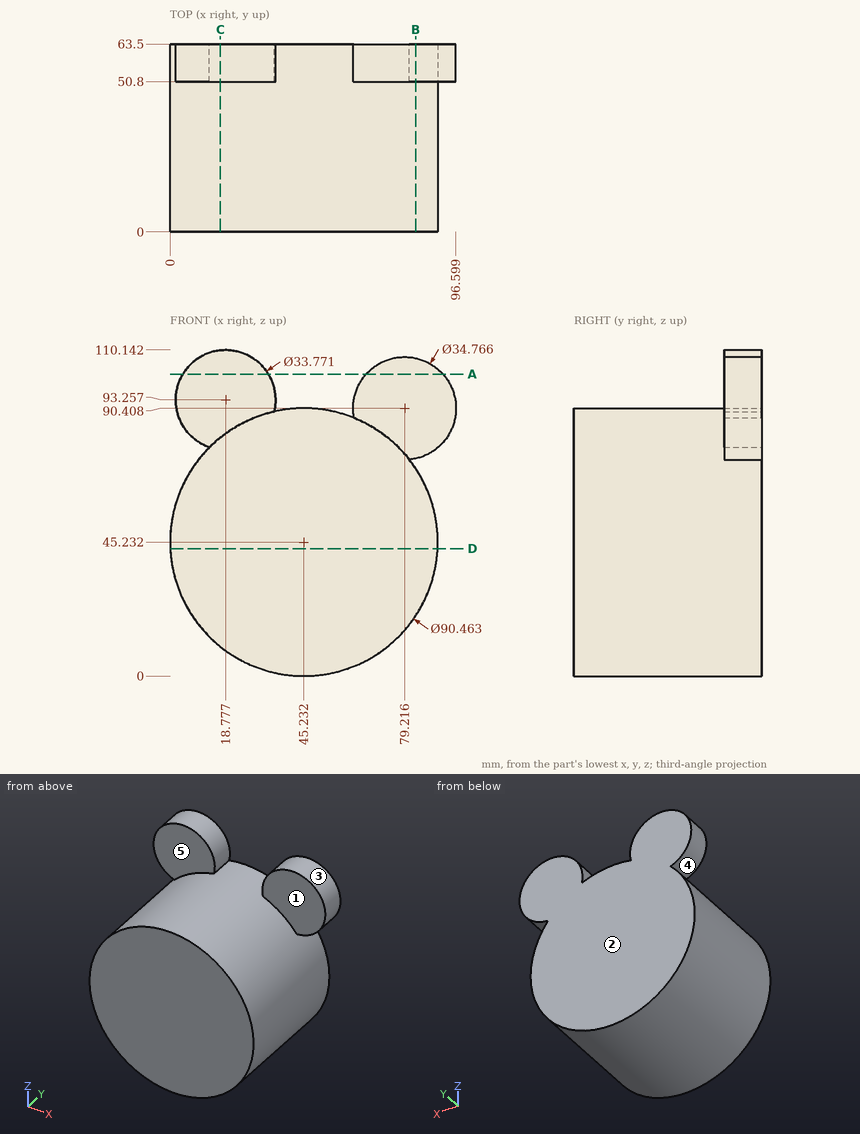
Geometry: see drawing. Coordinates: mm, zero at the bounding-box minimum. A direction names the side the tool comes from. Give positions to 0.01 mm unless a question says otherwise; leave off trailing zeros. Order: outer loops, then holes, each group sorted by start corner. A loop starts at its lowest first (then second) coordinate and runs counter-clockwise, first axis right, second up.
1. Pin query (flat end, axial travel): pin 1 Ø17.5 at (x, z) = (78, 93.5) entering from -Y; pin 2 Ø5 at (x, z) = (53.5, 80.5) entering from -Y; pin 3 Ø8 at (x, y) = (83, 12.5) entering from -Z; pin 4 Ø8 at (x, y) = (86.5, 47) entering from +Z. Return the tip coordinate at first contact, or that it passes through.
Computed:
pin 1: stops at y = 50.8
pin 2: stops at y = 0
pin 3: stops at z = 15.14
pin 4: stops at z = 106.71
2. Cut plane A-A (z = 102). Return loops of the section in (x, y).
Computed:
outline: (4.33, 50.8) - (33.22, 50.8) - (33.22, 63.5) - (4.33, 63.5) - close; (66.26, 50.8) - (92.17, 50.8) - (92.17, 63.5) - (66.26, 63.5) - close
3. Line query: probe 1 along Y at (x, z) = (83, 100); probe 2 along Z at (x, y) = (64.5, 34) (1 decimal); probe 3 along X at (y, z) = (47, 49.5). Output: solid intervals per line, ascending.
Computed:
probe 1: y = 50.8 to 63.5
probe 2: z = 4.3 to 86.2
probe 3: x = 0.2 to 90.26
4. Cut plane B-B (x = 83). Return loops of the section in (y, z) (1 decimal), and give its area (3 significant figures).
Computed:
outline: (0, 20.3) - (63.5, 20.3) - (63.5, 70.1) - (0, 70.1) - close; (50.8, 73.4) - (63.5, 73.4) - (63.5, 107.4) - (50.8, 107.4) - close
area: 3,590 mm2
5. Cut plane D-D (z = 43). Return loops of the section in (x, y) (1 decimal).
Computed:
outline: (0.1, 0) - (90.4, 0) - (90.4, 63.5) - (0.1, 63.5) - close
6. Cut plane C-C (x = 17). Return loops of the section in (y, z), and give its area (3 significant figures).
Computed:
outline: (0, 9.89) - (63.5, 9.89) - (63.5, 110.05) - (50.8, 110.05) - (50.8, 80.57) - (0, 80.57) - close
area: 4,860 mm2
7. Set-up query: the marked faces 1 and 2. Return all of +Z, -Z, +X, -X, +Y, -Y with unobstructed straight access to the full face (end or side cutting, diameter ignored); none if empty.
Computed:
face 1: +Z, +X, -Y
face 2: +Z, -Z, +X, -X, +Y
8. Draft query along X for the marked faces 3, 4 and 5. Return one class per face: released by +X, released by -X, zero draft, split by the parting line, or undercut.
Computed:
face 3: undercut
face 4: undercut
face 5: zero draft
